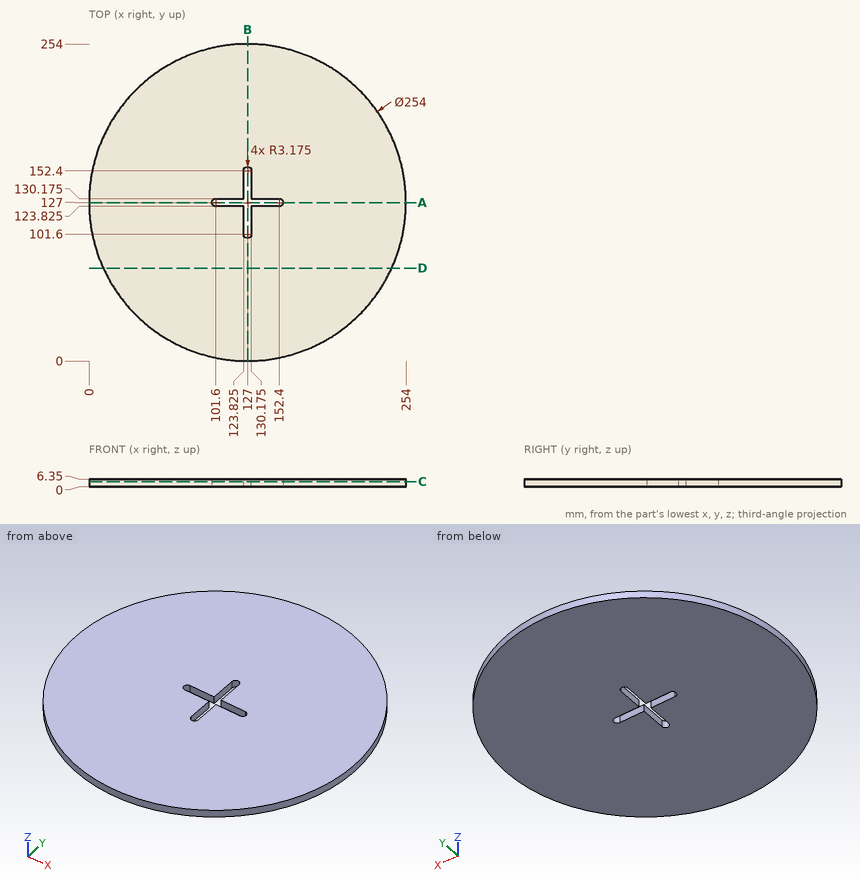
Could you check a few things on this drawing? It's one solid part, dimensions in mm from its lowest x, y, z. Coordinates: 2 decimals unless noted, no trailing zeros. Order: outer loops, then holes, each group sorted by start corner. A loop starts at its lowest first (then second) coordinate and runs counter-clockwise, first axis right, second up.
1) Imagine slicing it at D-D on y = 74.5. List the corners of the cut face in (x, z) for me.
2) Will these pins go through, and if not, where does the flat tip stop? pin 1 (1.9 mm diameter, centred on y = 107.5, z = 1.5, fed in from -X); pin 2 (1.9 mm diameter, centred on y = 144, z = 2.5, fed in from +X); pin 3 (1 mm diameter, centred on x = 185.5, z = 2.5, fed in from +Y).
3) Imagine slicing it at C-C on z = 4.25. List the corners of the cut face in (x, y) for me (3 decimals).
4) I need wall thicknesses on line 1 (X direction, y = 100.5, z = 3); line 2 (Y direction, x = 150.5, z = 5.5) (3 decimals); line 3 (X direction, y = 119.5, z = 1.5) (3 decimals). Which ranges of each line are inside material? Lowest first, please.
5) Imagine slicing it at A-A on y = 127. List the corners of the cut face in (x, z) for me (3 decimals), and give its area (3 significant figures).
Response values:
1. outline: (11.36, 0) - (242.64, 0) - (242.64, 6.35) - (11.36, 6.35) - close
2. pin 1: stops at x = 1.36
2. pin 2: stops at x = 252.98
2. pin 3: stops at y = 239.98
3. outline: circle Ø254 at (127, 127); hole (101.6, 123.825) - (123.825, 123.825) - (123.825, 101.6) arc R3.175 ccw to (130.175, 101.6) - (130.175, 123.825) - (152.4, 123.825) arc R3.175 ccw to (152.4, 130.175) - (130.175, 130.175) - (130.175, 152.4) arc R3.175 ccw to (123.825, 152.4) - (123.825, 130.175) - (101.6, 130.175) arc R3.175 ccw to start
4. line 1: x = 2.8 to 124.02, 129.98 to 251.2
4. line 2: y = 2.193 to 123.825, 130.175 to 251.807
4. line 3: x = 0.222 to 123.825, 130.175 to 253.778
5. outline: (0, 0) - (98.425, 0) - (98.425, 6.35) - (0, 6.35) - close; (155.575, 0) - (254, 0) - (254, 6.35) - (155.575, 6.35) - close
5. area: 1,250 mm2
